Work out the finished part from the listing and answer in its coordinate system (mm). Coordinates: 2 decimals unless noted, no trailing zeros. Order: outer loops, then holes, each group sorted by start corner. A loop starts at its lowest first (then second) coordinate and runs counter-clockwise, first axis right, second up. Notation, with made-up numbers: (42, 62.25) - (97, 62.25) arc R21 ccw to (97, 84.25) - close; hole circle Ø9 at (-27.5, 88). An arc over 180 degrees is marked (long way). Answer as a JSON object with one key per item and string values. Group by question number.
1) Section C-C (x = 52) is taken. Give the vertices of the cut face in (y, z), plus the area to 3 significant figures.
2) Find the intervals of material crossed by line 1 along Y through (x, z) = (-52.5, 1.2); line 2 along Y through (x, z) = (-14, 1.35); line 3 along Y through (x, z) = (-27, 1.8), in increasing order.
3) Section B-B (z = 1.95) is taken. Count the separate pieces of the cut face and the enclosed holes in it, plus the area to 3 significant figures.
4) Section A-A (y = 0) is taken. Give the vertices of the cut face in (x, z), plus the area to 3 significant figures.
5) Each of these flat-tipped pins is pushed along its axis until it touches: P1, Ø1.5, axis at y = -2, z = 2, coming from the +X side; P2, Ø0.9, axis at x = -38.5, z = 1.5, coming from the -Y side. Where does it stop, or does it pass through?
from build123d import *

# Parameters (mm, degrees)
BOSS_EXTRUDE1_DEPTH = 3
SKETCH2_R           = 10
CUT_EXTRUDE1_DEPTH  = 115.057003292


with BuildPart() as part:
    # Sketch1 → Boss-Extrude1 (new body)
    with BuildSketch(Plane.XY):
        Polygon((-50, 30), (-90, 30), (-90, 10), (-87, 10), (-87, -10), (-90, -10), (-90, -30), (-50, -30), (-50, -27), (-10, -27), (-10, -30), (30, -30), (30, -27), (70, -27), (70, -30), (71.400928912, -30), (110, -30), (110, -10), (107, -10), (107, 10), (110, 10), (110, 30), (71.400928912, 30), (70, 30), (70, 27), (30, 27), (30, 30), (-10, 30), (-10, 27), (-50, 27), align=None)
    extrude(amount=BOSS_EXTRUDE1_DEPTH)

    # Sketch2 → Cut-Extrude1 (cut, through all)
    with BuildSketch(Plane.XY.offset(3)):
        with Locations((-50, 0)):
            Circle(SKETCH2_R)
        with Locations((-10, 0)):
            Circle(SKETCH2_R)
        with Locations((30, 0)):
            Circle(SKETCH2_R)
        with Locations((70, 0)):
            Circle(SKETCH2_R)
    extrude(amount=-CUT_EXTRUDE1_DEPTH, mode=Mode.SUBTRACT)


solid = part.part
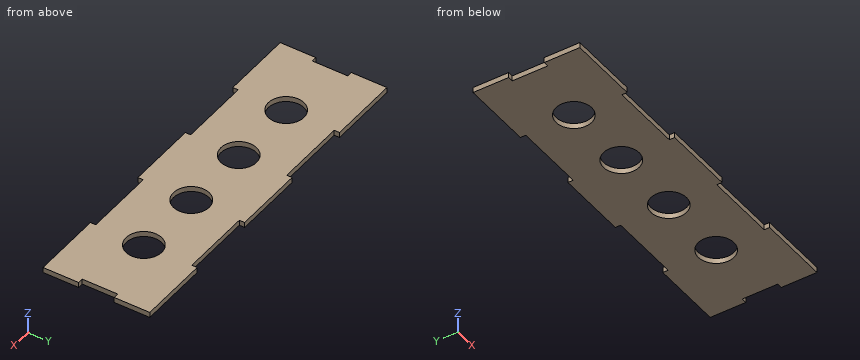
Report:
{
 "1": {"outline": "(-27, 0) - (27, 0) - (27, 3) - (-27, 3) - close", "area": "162 mm²"},
 "2": {"line 1": "y = -30 to -9.68, 9.68 to 30", "line 2": "y = -27 to -9.17, 9.17 to 27", "line 3": "y = -27 to 27"},
 "3": {"separate pieces": "1", "enclosed holes": "4", "area": "10,100 mm²"},
 "4": {"outline": "(-87, 0) - (-60, 0) - (-60, 3) - (-87, 3) - close; (-40, 0) - (-20, 0) - (-20, 3) - (-40, 3) - close; (0, 0) - (20, 0) - (20, 3) - (0, 3) - close; (40, 0) - (60, 0) - (60, 3) - (40, 3) - close; (80, 0) - (107, 0) - (107, 3) - (80, 3) - close", "area": "342 mm²"},
 "5": {"P1": "stops at x = 107", "P2": "stops at y = -27"}
}
